The drawing under review shows one solid part. Ordinate dimensions are in mm from its lowest x, y, z. A direction names the side the tool comes from. Give positions to 0.01 mm unless a question says otherwise; leave off trailing zeros. Loops run counter-clockwise (first coordinate to the right, second up) from the corner with the lowest first, then second, coordinate; pieces in that order, holes last. Notation, with made-up numbers: (11, -10.5) -> (29, -10.5) arc R17 ccw to (29, 5.5) -> close; hole circle Ø9 at (11, -15). An arc over 180 degrees is marked (long way). Answer in a Markdown table with one row per item. Add a question column.
(1) For pin 1 (2.5 mm diameter, centred on x = 8, y = 26.5, fed in from +Z); pin 2 (2 mm diameter, centred on x = 15.5, z = 0.5, fed in from -Y), all flat-tipped, find the tip position at first contact; note any pin that passes through.
(2) For the marked faces 1, 2 and 3, list the 3-axis set-ups (+Z, -Z, +X, -X, +Y, -Y) from which the entire face can be reached by the end or side of a thin tool; tool diameter is ignored.
(3) Consider section A-A on y = 19. Write out the cut boundary in (x, z), then the cut area to 3 significant figures.
(4) Consider section D-D on z = 1.1. Write out the cut boundary in (x, y), then the cut area to 3 significant figures.
(5) Draft analysis for pull direction Y (two halves, no side actions). For the marked faces 4, 5 and 6, state which applies: +Y half, -Y half, draft (parallel to the pull), parting line (faces both ways), or undercut.
(6) For line 1 (Y direction, x = 8, z = 2.8); line 2 (X direction, y = 9.5, z = 0.9); line 3 (Y direction, x = 23.5, z = 0.55), list the stretches that pass through material, from the lowest coordinate up.
(7) Consider section B-B on x = 8. Write out the cut boundary in (y, z).
(8) Consider section C-C on y = 26.5. Write out the cut boundary in (x, z).
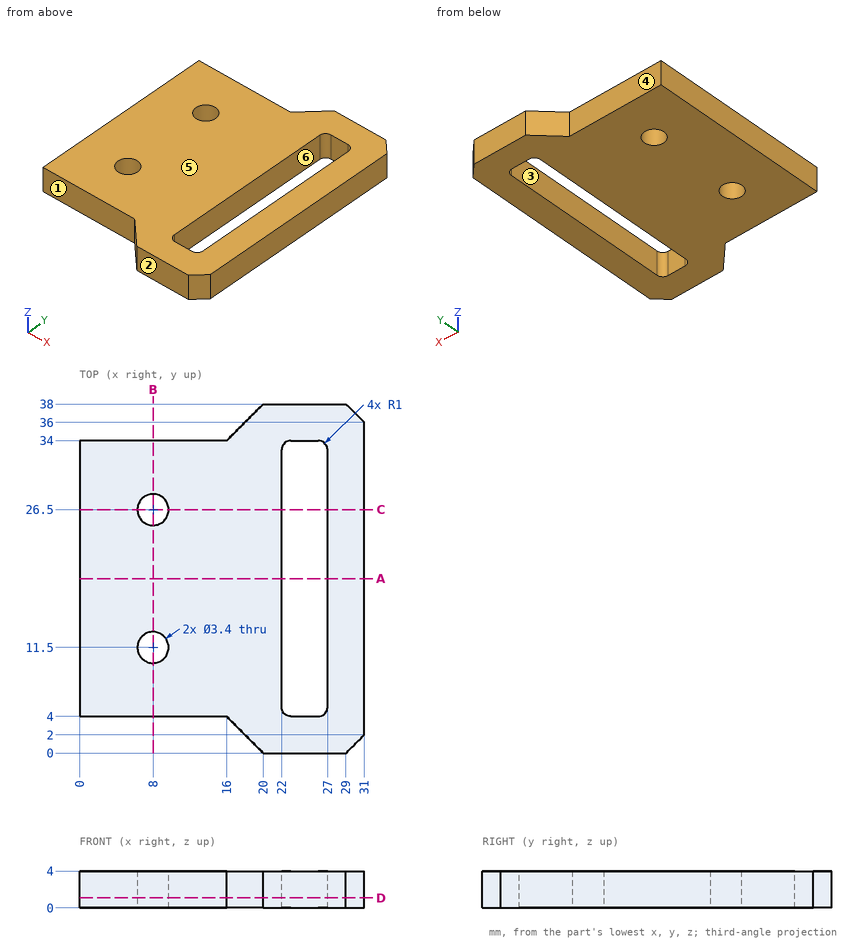
Values follow:
| question | item | result |
|---|---|---|
| 1 | pin 1 | through |
| 1 | pin 2 | y = 3.5 |
| 2 | face 1 | +Z, -Z, -X, -Y |
| 2 | face 2 | +Z, -Z, +X, -X, -Y |
| 2 | face 3 | +Z, -Z |
| 3 | outline | (0, 0) -> (22, 0) -> (22, 4) -> (0, 4) -> close; (27, 0) -> (31, 0) -> (31, 4) -> (27, 4) -> close |
| 3 | area | 104 mm2 |
| 4 | outline | (0, 4) -> (16, 4) -> (20, 0) -> (29, 0) -> (31, 2) -> (31, 36) -> (29, 38) -> (20, 38) -> (16, 34) -> (0, 34) -> close; hole circle Ø3.4 at (8, 11.5); hole circle Ø3.4 at (8, 26.5); hole (22, 5) arc R1 ccw to (23, 4) -> (26, 4) arc R1 ccw to (27, 5) -> (27, 33) arc R1 ccw to (26, 34) -> (23, 34) arc R1 ccw to (22, 33) -> close |
| 4 | area | 863 mm2 |
| 5 | face 4 | +Y half |
| 5 | face 5 | draft |
| 5 | face 6 | undercut |
| 6 | line 1 | 4 to 9.8, 13.2 to 24.8, 28.2 to 34 |
| 6 | line 2 | 0 to 22, 27 to 31 |
| 6 | line 3 | 0 to 4, 34 to 38 |
| 7 | outline | (4, 0) -> (9.8, 0) -> (9.8, 4) -> (4, 4) -> close; (13.2, 0) -> (24.8, 0) -> (24.8, 4) -> (13.2, 4) -> close; (28.2, 0) -> (34, 0) -> (34, 4) -> (28.2, 4) -> close |
| 8 | outline | (0, 0) -> (6.3, 0) -> (6.3, 4) -> (0, 4) -> close; (9.7, 0) -> (22, 0) -> (22, 4) -> (9.7, 4) -> close; (27, 0) -> (31, 0) -> (31, 4) -> (27, 4) -> close |
